from build123d import *

# Parameters (mm, degrees)
F0_R     = 76.2
F1_DEPTH = 76.2
F2_R     = 76.2
F3_R     = 76.19999


# Not quite as in the source:
# - a fillet or chamfer is up to 0.001 mm smaller than in the source, because OpenCascade refuses the exact size


with BuildPart() as f1:
    # F0 (on Front) → F1 (new body, symmetric)
    with BuildSketch(Plane.XZ):
        Circle(F0_R)
    extrude(amount=F1_DEPTH, both=True)

    # F2
    f2_edges = [f1.edges().sort_by_distance(p)[0] for p in [
        (-76.2, -76.2, 0),
    ]]
    fillet(f2_edges, radius=F2_R)

    # F3 (radius 76.2 in the source; OpenCascade refuses exactly that, so slightly less here)
    f3_edges = [f1.edges().sort_by_distance(p)[0] for p in [
        (-76.2, 76.2, 0),
    ]]
    fillet(f3_edges, radius=F3_R)


solid = f1.part
Verification items for the finished model (mm, model axes). Give positions to 0.01 mm unless a question says otherwise; leave off trailing zeros. Loops run counter-clockwise (first coordinate to the right, second up) from the corner with the lowest first, then second, coordinate; pieces in that order, holes last. Notation, with made-up numbers: (30.5, 84.5) - (76.5, 84.5) arc R19 cw to (76.5, 98.5) - close; hole circle Ø8 at (-1.5, -37). An arc over 180 degrees is marked (long way). Write item = value, one per line. Start each with the question number.
Q1. Cross-section at A-A, the plane y = -7.5. Enter the section's corners in (x, z), and give its area (3 significant figures).
Q2. Depth check by flat-ended pin: P1, Ø5, axis at x = -37.5, z = 36.5, coming from the -Y side; P2, Ø5, axis at x = 15, y = -37, coming from the -Z side; P3, Ø1.5, axis at x = -43.5, z = -48.5, coming from the -Y side. Enter the tip coordinate at first touch or a pass-through.
Q3. Cross-section at B-B, the plane y = -55.5. Enter the section's corners in (x, z).
Q4. Thickness scan on line 1 (X direction, y = -16.5, z = 3.5); line 2 (Y direction, x = -20.5, z = -2.5); line 3 (X direction, y = -26, z = -44). Record the ranges inside material, lowest first.
Answer key:
q1.outline = circle Ø151.66 at (0, 0)
q1.area = 18,100 mm^2
q2.P1 = -57.65
q2.P2 = -66.38
q2.P3 = -40.73
q3.outline = circle Ø104.43 at (0, 0)
q4.line_1 = -74.31 to 74.31
q4.line_2 = -73.35 to 73.35
q4.line_3 = -56.52 to 56.52
